Can you work these out from the model? Positions are in its coordinate system, mm. Face numbers are marked on the shaded views. A direction names the side the tool comes from. Round coordinates to 2 decimals unless told otherwise and drop trailing zeros. Loops run counter-clockwise (first coordinate to the right, second up) from the corner with the lowest first, then second, coordinate; pieces in that order, holes last.
(1) Thinking about a two-plate mould opening in X: for the marked faces 4, 5 and 6, which applies, released by +X, released by -X, zero draft, split by the parting line, or undercut?
(2) I want a section at B-B on z = 2. Write out the boundary of the cut face in (x, y).
(3) I want a section at A-A on x = 0. Write out the boundary of the cut face in (y, z).
(4) If I drill on line 1 along X through (y, z) = (0, 3); line 2 along X through (y, z) = (0, -10); line 3 along Y through (x, z) = (0, -8), over which ranges is the centre line in solid material (lowest first)?
(5) Will these pins go through, and if not, where does the flat tip stop? pin 1 Ø10 at (y, z) = (-17, 3) entering from +X; pin 2 Ø1 at (y, z) = (2, -5.5) entering from -X; pin 3 Ø2 at (y, z) = (-33, -4) entering from -X.
(6) Which directions (+Z, -Z, +X, -X, +Y, -Y) give clear straight access to the entire face, cutting with the end or side of a thin tool? Please do the marked faces 1, 2 and 3.
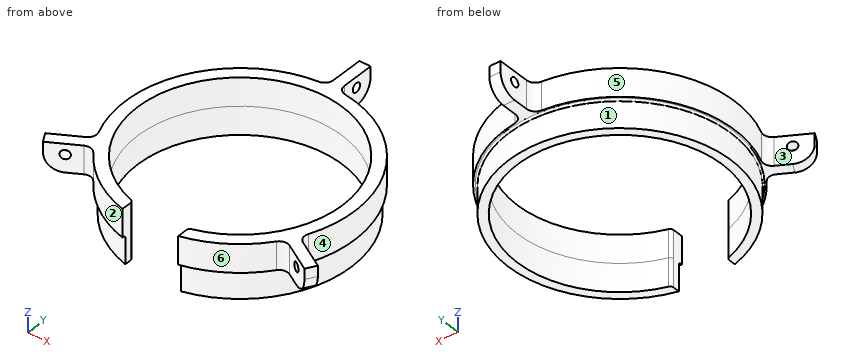
from build123d import *

# Parameters (mm, degrees)
SKETCH_R              = 88.5
SKETCH_R_2            = 58.5
PAD_DEPTH             = 16
POCKET_DEPTH          = 517.654267
POLARPATTERN_COUNT    = 3
SKETCH002_W           = 32
SKETCH002_H           = 137
POCKET001_DEPTH       = 16.001
SKETCH003_R           = 2.6
POCKET002_DEPTH       = 518.756447
POLARPATTERN001_COUNT = 3
PAD001_DEPTH          = 16
FILLET_R              = 1
FILLET001_R           = 2
FILLET002_R           = 10
FILLET003_R           = 5


with BuildPart() as part:
    # Sketch → Pad (new body)
    with BuildSketch(Plane.XY):
        Circle(SKETCH_R)
        Circle(SKETCH_R_2, mode=Mode.SUBTRACT)
    extrude(amount=PAD_DEPTH)

    # Sketch001 (on Face4 of Pad) → Pocket (cut, through all)
    with BuildSketch(Plane.XY.offset(16)):
        with BuildLine():
            ThreePointArc((58.256928, -29.939611), (56.724664, 32.75), (3.2, 65.421785))
            Line((3.2, 192.421785), (3.2, 65.421785))
            ThreePointArc((168.242154, -93.439611), (166.665196, 96.224196), (3.2, 192.421785))
            Line((58.256928, -29.939611), (168.242154, -93.439611))
        make_face()
    pocket = extrude(amount=-POCKET_DEPTH, mode=Mode.SUBTRACT)

    # PolarPattern: Pocket ×3 about axis
    polarpattern_axis = Axis((0, 0, 16), (0, 0, 1))
    for i in range(1, POLARPATTERN_COUNT):
        add(pocket.rotate(polarpattern_axis, i * 360 / POLARPATTERN_COUNT), mode=Mode.SUBTRACT)

    # Sketch002 (on Face4 of PolarPattern) → Pocket001 (cut, through all)
    with BuildSketch(Plane.XY.offset(16)):
        with Locations((0, -68.5)):
            Rectangle(SKETCH002_W, SKETCH002_H)
    extrude(amount=-POCKET001_DEPTH, mode=Mode.SUBTRACT)

    # Sketch003 (on Face5 of Pocket001) → Pocket002 (cut, through all)
    with BuildSketch(Plane.YZ.offset(3.2)):
        with Locations((78.442128, 10)):
            Circle(SKETCH003_R)
    pocket002 = extrude(amount=-POCKET002_DEPTH, mode=Mode.SUBTRACT)

    # PolarPattern001: Pocket002 ×3 about axis
    polarpattern001_axis = Axis((0, 0, 0), (0, 0, 1))
    for i in range(1, POLARPATTERN001_COUNT):
        add(pocket002.rotate(polarpattern001_axis, i * 360 / POLARPATTERN001_COUNT), mode=Mode.SUBTRACT)

    # Sketch004 (on Face2 of PolarPattern001) → Pad001 (join)
    with BuildSketch(Plane(origin=(0, 0, 0), x_dir=(1, 0, 0), z_dir=(0, 0, -1))):
        with BuildLine():
            ThreePointArc((-16, 56.269441), (0, -58.5), (16, 56.269441))
            Line((16, 61.515746), (16, 56.269441))
            ThreePointArc((-16, 61.515746), (0, -63.562465), (16, 61.515746))
            Line((-16, 61.515746), (-16, 56.269441))
        make_face()
    extrude(amount=PAD001_DEPTH)

    # Fillet
    fillet_edges = [part.edges().sort_by_distance(p)[0] for p in [
        (0, 63.562465, 0),
    ]]
    fillet(fillet_edges, radius=FILLET_R)

    # Fillet001
    fillet001_edges = [part.edges().sort_by_distance(p)[0] for p in [
        (-16, -56.269441, -8),
        (-16, -56.269441, 8),
        (16, -56.269441, -8),
        (16, -56.269441, 8),
    ]]
    fillet(fillet001_edges, radius=FILLET001_R)

    # Fillet002
    fillet002_edges = [part.edges().sort_by_distance(p)[0] for p in [
        (-76.643248, -44.25, 0),
        (76.643248, -44.25, 0),
        (0, 88.5, 0),
    ]]
    fillet(fillet002_edges, radius=FILLET002_R)

    # Fillet003
    fillet003_edges = [part.edges().sort_by_distance(p)[0] for p in [
        (58.256928, -29.939611, 8),
        (55.056928, -35.482174, 8),
        (-55.056928, -35.482174, 8),
        (-58.256928, -29.939611, 8),
        (-3.2, 65.421785, 8),
        (3.2, 65.421785, 8),
    ]]
    fillet(fillet003_edges, radius=FILLET003_R)


solid = part.part
Filled sheet:
1. face 4: released by +X
1. face 5: released by -X
1. face 6: undercut
2. outline: (-74.73, -39.45) arc R84.5 ccw to (-71.53, -44.99) - (-59.04, -37.78) arc R5 cw to (-52.53, -39.13) arc R65.5 ccw to (-16, -63.52) - (-16, -57.76) arc R2 ccw to (-17.4, -55.85) arc R58.5 cw (long way) to (17.4, -55.85) arc R2 ccw to (16, -57.76) - (16, -63.52) arc R65.5 ccw to (52.53, -39.13) arc R5 cw to (59.04, -37.78) - (71.53, -44.99) arc R84.5 ccw to (74.73, -39.45) - (62.24, -32.24) arc R5 cw to (60.15, -25.93) arc R65.5 ccw to (7.62, 65.06) arc R5 cw to (3.2, 70.02) - (3.2, 84.44) arc R84.5 ccw to (-3.2, 84.44) - (-3.2, 70.02) arc R5 cw to (-7.62, 65.06) arc R65.5 ccw to (-60.15, -25.93) arc R5 cw to (-62.24, -32.24) - close
3. outline: (58.5, -16) - (63.56, -16) - (63.56, -1) arc R1 cw to (64.56, 0) - (78.5, 0) arc R10 ccw to (88.5, 10) - (88.5, 16) - (58.5, 16) - close; hole circle Ø5.2 at (78.44, 10)
4. line 1: x = -65.5 to -58.5, 58.5 to 65.5
4. line 2: x = -63.56 to -58.5, 58.5 to 63.56
4. line 3: y = 58.5 to 63.56
5. pin 1: stops at x = 64.39
5. pin 2: stops at x = -63.54
5. pin 3: stops at x = -54.92
6. face 1: -Z
6. face 2: +Z, -Z, -Y
6. face 3: +Z, -Z, -X
